Work out the finished part from the listing and answer in its coordinate system (mm). A direction names the side the tool comes from. Round coordinates to 2 decimals unless told otherwise and drop trailing zeros. Write each loop counter-clockwise with the first axis right and the second up, starting at its lowest first coordinate (ties: lowest second). Pieces come first, ordered by that corner, then holes. Notation, with made-up numbers: (10, 27.5) -> (69, 27.5) arc R23 ccw to (69, 47.5) -> close; hole circle Ø10 at (63.5, 45). An arc over 180 degrees is marked (long way). Answer as a JSON object with one key per item and string values. Group by question number.
from build123d import *

# Parameters (mm, degrees)
SKETCH_1_R           = 49
SKETCH_1_R_2         = 37.5
SKETCH_1_R_3         = 2
EXTRUDE_1_DEPTH      = 15.5
EXTRUDE_START        = 15.5
SKETCH_1_3_R         = 49
SKETCH_1_3_R_2       = 2
EXTRUDE_2_DEPTH      = 4
CUT_EXTRUDE_START    = -8
SKETCH_2_W           = 31.667504192
SKETCH_2_H           = 35
CUT_EXTRUDE_1_DEPTH  = 8.5
SKETCH_4_R           = 3.25
CUT_EXTRUDE_3_DEPTH  = 15.5
CUT_EXTRUDE_START_2  = -13.5
SKETCH_6_R           = 49
SKETCH_6_R_2         = 41
CUT_EXTRUDE_7_DEPTH  = 13.5
SKETCH_8_R           = 2
CUT_EXTRUDE_9_DEPTH  = 16.5
SKETCH_7_W           = 30
SKETCH_7_H           = 31
CUT_EXTRUDE_11_DEPTH = 2
SKETCH_10_R          = 1
CUT_EXTRUDE_13_DEPTH = 2
SKETCH_12_W          = 94.768438907
SKETCH_12_H          = 47.5
CUT_EXTRUDE_14_DEPTH = 13.5
CHAMFER_1_SIZE       = 3
CHAMFER_2_SIZE       = 3
CHAMFER_3_SIZE       = 3


with BuildPart() as part:
    # 스케치1 → 보스-돌출1 (new body)
    with BuildSketch(Plane(origin=(0, 0, 0), x_dir=(1, 0, 0), z_dir=(0, 1, 0))):
        with Locations(Location((0, 0, 0), (0, 0, 270))):
            Circle(SKETCH_1_R)
        with Locations(Location((0, 0, 0), (0, 0, 270))):
            Circle(SKETCH_1_R_2, mode=Mode.SUBTRACT)
        with Locations(Location((-43.466662183, 11.64685703, 0), (0, 0, 270))):
            Circle(SKETCH_1_R_3, mode=Mode.SUBTRACT)
        with Locations(Location((-11.64685703, 43.466662183, 0), (0, 0, 270))):
            Circle(SKETCH_1_R_3, mode=Mode.SUBTRACT)
        with Locations(Location((31.819805153, 31.819805153, 0), (0, 0, 270))):
            Circle(SKETCH_1_R_3, mode=Mode.SUBTRACT)
        with Locations(Location((43.466662183, -11.64685703, 0), (0, 0, 270))):
            Circle(SKETCH_1_R_3, mode=Mode.SUBTRACT)
        with Locations(Location((11.64685703, -43.466662183, 0), (0, 0, 270))):
            Circle(SKETCH_1_R_3, mode=Mode.SUBTRACT)
        with Locations(Location((-31.819805153, -31.819805153, 0), (0, 0, 270))):
            Circle(SKETCH_1_R_3, mode=Mode.SUBTRACT)
    extrude(amount=EXTRUDE_1_DEPTH)

    # 스케치1<3> → 보스-돌출2 (add)
    with BuildSketch(Plane(origin=(0, 0, 0), x_dir=(1, 0, 0), z_dir=(0, 1, 0)).offset(EXTRUDE_START)):
        with Locations(Location((0, 0, 0), (0, 0, 270))):
            Circle(SKETCH_1_3_R)
        with Locations(Location((-43.466662183, 11.64685703, 0), (0, 0, 270))):
            Circle(SKETCH_1_3_R_2, mode=Mode.SUBTRACT)
        with Locations(Location((-11.64685703, 43.466662183, 0), (0, 0, 270))):
            Circle(SKETCH_1_3_R_2, mode=Mode.SUBTRACT)
        with Locations(Location((31.819805153, 31.819805153, 0), (0, 0, 270))):
            Circle(SKETCH_1_3_R_2, mode=Mode.SUBTRACT)
        with Locations(Location((43.466662183, -11.64685703, 0), (0, 0, 270))):
            Circle(SKETCH_1_3_R_2, mode=Mode.SUBTRACT)
        with Locations(Location((11.64685703, -43.466662183, 0), (0, 0, 270))):
            Circle(SKETCH_1_3_R_2, mode=Mode.SUBTRACT)
        with Locations(Location((-31.819805153, -31.819805153, 0), (0, 0, 270))):
            Circle(SKETCH_1_3_R_2, mode=Mode.SUBTRACT)
    extrude(amount=EXTRUDE_2_DEPTH)

    # 스케치2 → 컷-돌출1 (cut)
    with BuildSketch(Plane(origin=(0, 19.5, 0), x_dir=(1, 0, 0), z_dir=(0, 1, 0)).offset(CUT_EXTRUDE_START)):
        with Locations((-49, 0)):
            Rectangle(SKETCH_2_W, SKETCH_2_H)
    extrude(amount=-CUT_EXTRUDE_1_DEPTH, mode=Mode.SUBTRACT)

    # 스케치4 → 컷-돌출3 (cut)
    with BuildSketch(Plane(origin=(0, 19.5, 0), x_dir=(1, 0, 0), z_dir=(0, 1, 0))):
        with Locations(Location((-11.64685703, 43.466662183, 0), (0, 0, 270))):
            Circle(SKETCH_4_R)
        with Locations(Location((31.819805153, 31.819805153, 0), (0, 0, 270))):
            Circle(SKETCH_4_R)
        with Locations(Location((43.466662183, -11.64685703, 0), (0, 0, 270))):
            Circle(SKETCH_4_R)
        with Locations(Location((11.64685703, -43.466662183, 0), (0, 0, 270))):
            Circle(SKETCH_4_R)
        with Locations(Location((-31.819805153, -31.819805153, 0), (0, 0, 270))):
            Circle(SKETCH_4_R)
        with Locations(Location((-43.466662183, 11.64685703, 0), (0, 0, 270))):
            Circle(SKETCH_4_R)
    extrude(amount=-CUT_EXTRUDE_3_DEPTH, mode=Mode.SUBTRACT)

    # 스케치6 → 컷-돌출7 (cut)
    with BuildSketch(Plane(origin=(0, 19.5, 0), x_dir=(1, 0, 0), z_dir=(0, 1, 0)).offset(CUT_EXTRUDE_START_2)):
        with Locations(Location((0, 0, 0), (0, 0, 159.075167572))):
            Circle(SKETCH_6_R)
        with Locations(Location((0, 0, 0), (0, 0, 270))):
            Circle(SKETCH_6_R_2, mode=Mode.SUBTRACT)
    extrude(amount=CUT_EXTRUDE_7_DEPTH, mode=Mode.SUBTRACT)

    # 스케치8 → 컷-돌출9 (cut)
    with BuildSketch(Plane(origin=(0, 19.5, 0), x_dir=(1, 0, 0), z_dir=(0, 1, 0))):
        with Locations(Location((0, -7, 0), (0, 0, 270))):
            Circle(SKETCH_8_R)
        with Locations(Location((10.392304845, -13, 0), (0, 0, 270))):
            Circle(SKETCH_8_R)
        with Locations(Location((10.392304845, -25, 0), (0, 0, 270))):
            Circle(SKETCH_8_R)
        with Locations(Location((0, -31, 0), (0, 0, 270))):
            Circle(SKETCH_8_R)
        with Locations(Location((-10.392304845, -25, 0), (0, 0, 270))):
            Circle(SKETCH_8_R)
        with Locations(Location((-10.392304845, -13, 0), (0, 0, 270))):
            Circle(SKETCH_8_R)
    extrude(amount=-CUT_EXTRUDE_9_DEPTH, mode=Mode.SUBTRACT)

    # 스케치7 → 컷-돌출11 (cut)
    with BuildSketch(Plane(origin=(0, 19.5, 0), x_dir=(1, 0, 0), z_dir=(0, 1, 0))):
        with Locations((0, -19)):
            Rectangle(SKETCH_7_W, SKETCH_7_H)
    extrude(amount=-CUT_EXTRUDE_11_DEPTH, mode=Mode.SUBTRACT)

    # 스케치10 → 컷-돌출13 (cut)
    with BuildSketch(Plane(origin=(0, 19.5, 0), x_dir=(1, 0, 0), z_dir=(0, 1, 0))):
        with Locations((-15, -3.5)):
            Circle(SKETCH_10_R)
        with Locations((15, -3.5)):
            Circle(SKETCH_10_R)
        with Locations((15, -34.5)):
            Circle(SKETCH_10_R)
        with Locations((-15, -34.5)):
            Circle(SKETCH_10_R)
    extrude(amount=-CUT_EXTRUDE_13_DEPTH, mode=Mode.SUBTRACT)

    # 스케치12 → 컷-돌출14 (cut)
    with BuildSketch(Plane(origin=(0, 19.5, 0), x_dir=(1, 0, 0), z_dir=(0, 1, 0))):
        with Locations((1.615780546, 25.25)):
            Rectangle(SKETCH_12_W, SKETCH_12_H)
    extrude(amount=-CUT_EXTRUDE_14_DEPTH, mode=Mode.SUBTRACT)

    # 모따기1
    chamfer_1_edges = [part.edges().sort_by_distance(p)[0] for p in [
        (0, 19.5, -1.5),
    ]]
    chamfer(chamfer_1_edges, length=CHAMFER_1_SIZE)

    # 모따기2
    # the kernel refuses this chamfer: 3 mm, written as the material it takes off along each edge
    with BuildSketch(Plane(origin=(0, 6, 0), x_dir=(-0.978595972723543, 0, -0.20579096717121165), z_dir=(-0.20579096717121165, 0, 0.978595972723543))) as chamfer_2_piece_1:
        Polygon((49 - CHAMFER_2_SIZE, 0), (49, CHAMFER_2_SIZE), (49, 0), align=None)
    revolve(axis=Axis((0, 6, 0), (0, -1, 0)), revolution_arc=258.124194574, mode=Mode.SUBTRACT)
    with BuildSketch(Plane(origin=(0, 6, 0), x_dir=(-0.9785036629782533, 0, 0.20622943906760932), z_dir=(-0.20622943906760932, 0, -0.9785036629782533))) as chamfer_2_piece_2:
        Polygon((49 - CHAMFER_2_SIZE, 0), (49, -CHAMFER_2_SIZE), (49, 0), align=None)
    revolve(axis=Axis((0, 6, 0), (0, 1, 0)), revolution_arc=78.098521288, mode=Mode.SUBTRACT)

    # 모따기3
    # the kernel refuses this chamfer: 3 mm, written as the material it takes off along each edge
    with BuildSketch(Plane(origin=(0, 19.5, 0), x_dir=(0.9884903448479317, 0, -0.15128396525216095), z_dir=(-0.15128396525216095, 0, -0.9884903448479317))) as chamfer_3_piece_1:
        Polygon((41, CHAMFER_3_SIZE), (41 - CHAMFER_3_SIZE, 0), (41, 0), align=None)
    revolve(axis=Axis((0, 19.5, 0), (0, -1, 0)), revolution_arc=197.402683099, mode=Mode.SUBTRACT)


solid = part.part
1) Each of these flat-tipped pins is pushed along its axis until it touches: P1, Ø2, axis at x = 33.5, z = -32, coming from the +Y side; P2, Ø6.5, axis at x = 10.39, z = 25, coming from the +Y side; P3, Ø5, axis at y = 6, z = -24.5, coming from the +X side; P4, Ø2.5, axis at x = 10.39, z = 13, coming from the +Y side. Where does it stop, or does it pass through?
2) A cutting plane is placed at A-A on z = 0. Determine the outline of the cut face in (x, y), plus the area to 3 significant figures.
3) A cutting plane is placed at C-C on y = 9.25. Determine the outline of the cut face in (x, z), plus the area to 3 significant figures.
4) For a pull along Y with two mould halves and no side action, classify faces 1 (the face through (11.744, 16.514, 23.526)), 2 (the face through (-30, 4, 30)), 3 (the face through (1, 15.5, 13)), 4 (the face through (-41, 3, 0)) as released by +Y, released by -Y, zero draft, split by the parting line, or undercut.
5) A cutting plane is placed at B-B on z = 25. State how many separate pieces and enclosed holes the cut face has, plus the area to 3 significant figures.
6) Straight lines are drawn through the part: L1, parallel to Z at x = 9.5, y = 16; L2, parallel to Z at x = 30, y = 2; L3, parallel to X at y = 3.75, z = 11.5. For each, find the intervals that lie inside material, in ascending order.
7) A tool of negligible diameter and unlimited length cuts with its end or side. For faces 5 (the face through (-38, 11.5, 8)), 6 (the face through (11.26, 5.92, 35.77)), 7 (the face through (-36.8, 6.4, 17.5)), from which of +Z, -Z, +X, -X, +Y, -Y can it reach the whole face along a straight path? Write none if from no direction.
Established:
{
 "1": {"P1": "stops at y = 4", "P2": "stops at y = 17.5", "P3": "stops at x = 42.19", "P4": "passes through"},
 "2": {"outline": "(-49, 0) -> (-37.5, 0) -> (-37.5, 3) -> (-49, 3) -> close; (-41, 11.5) -> (-37.5, 11.5) -> (-37.5, 15.5) -> (37.5, 15.5) -> (37.5, 0) -> (49, 0) -> (49, 3) -> (46, 6) -> (41, 6) -> (41, 16.5) -> (39.5, 18) -> (-39.5, 18) -> (-41, 16.5) -> close", "area": "349 mm²"},
 "3": {"outline": "(-37.08, 17.5) -> (-33.17, 17.5) arc R37.5 cw to (37.47, -1.5) -> (40.97, -1.5) arc R41 ccw to start", "area": "373 mm²"},
 "4": {"face 1": "zero draft", "face 2": "released by +Y", "face 3": "released by -Y", "face 4": "undercut"},
 "5": {"separate pieces": "3", "enclosed holes": "0", "area": "419 mm²"},
 "6": {"L1": "z = -1.5 to 11.21, 14.79 to 23.21, 26.79 to 39.88", "L2": "z = -38.74 to -32.65, -30.99 to -22.5, 22.5 to 38.74", "L3": "x = 35.69 to 41.47, 45.46 to 46.86"},
 "7": {"face 5": "-Z, -X", "face 6": "-Y", "face 7": "-X"}
}
